Verification items for the finished model (mm, model axes). A direction names the side the tool comes from. Give positions to 0.01 mm unless a question says otherwise; leave off trailing zeros. Order: outer loops, then holes, each group sorted by start corner. A loop starts at its lowest first (then second) coordinate and runs counter-clockwise, first axis right, second up. Notation, with made-up numbers: (-26.5, 39.25) -> (19.5, 39.25) arc R14 cw to (19.5, 48.25) -> close; hole circle Ø3 at (-4, 17.25). An arc over 180 degrees is marked (long way). Write each question's results on one line, items separated by ' | '. Start each with the question number.
1. Mould release check, pull along X, two halves, no side actions. Record for faces 6 (the face through (-11.247, 0.143, 4.324)), 7 (the face through (-12, 0, 3)), 8 (the face through (0, 0, -3)), 9 (the face through (9.6, 0.07, 1.28)): +X half, -X half, draft (parallel to the pull), parting line (faces both ways), or undercut.
2. Cross-section at B-B, the plane x = -7.5. Enter the section's corners in (y, z), then the cut area to 3 significant figures.
3. Depth check by flat-ended pin: pin 1 Ø2 at (y, z) = (0.5, -2) entering from -X; pin 2 Ø3.5 at (x, y) = (-8, 0) entering from +Z; pin 3 Ø2.5 at (x, z) = (0, -1.5) entering from +Y. Enter the tip coordinate at first touch or a pass-through.
4. Material ranges on L1, parallel to X at y = -1.75, z = 4.5; L2, parallel to Z at x = -5.25, y = 0.25; L3, parallel to Y at x = 2.75, z = -1, recorded low to high. Write a range as from..to.
5. Cross-section at C-C, the plane z = 4.5. Enter the section's corners in (x, y).
6. Cross-section at A-A, the plane y = 0. Enter the section's corners in (x, z).
7. Set-up check for faces 1 (the face through (-6.6, -1.4, 2.6)), 2 (the face through (5, 0, -1)), 3 (the face through (-5, 0, -1)), 4 (the face through (0, -3, -1)), 5 (the face through (0, 3, -1)): record each of +Z, -Z, +X, -X, +Y, -Y from which the full face is reachable in a straight line by a thin tool's end or side.
8. Cross-section at D-D, the plane x = 9.25. Enter the section's corners in (y, z).
from build123d import *

# Parameters (mm, degrees)
BOSS_EXTRU_1_DEPTH                                 = 6
CHAMBRAGE_POUR_VIS_T_TE_HEXAGONALE_M31_D           = 3.2
CHAMBRAGE_POUR_VIS_T_TE_HEXAGONALE_M31_CBORE_D     = 6.5
CHAMBRAGE_POUR_VIS_T_TE_HEXAGONALE_M31_CBORE_DEPTH = 3.4
ESQUISSE6_W                                        = 10
ESQUISSE6_H                                        = 8
BOSS_EXTRU_2_DEPTH                                 = 3
CHANFREIN1_SIZE                                    = 0.2
ENL_V_MAT_EXTRU_5_REACH                            = 20.466
ESQUISSE10_W                                       = 3
ESQUISSE10_H                                       = 1


with BuildPart() as part:
    # Esquisse1 → Boss.-Extru.1 (new body)
    with BuildSketch(Plane.XY):
        with BuildLine():
            Line((-8, 4), (8, 4))
            ThreePointArc((8, 4), (12, 0), (8, -4))
            Line((8, -4), (-8, -4))
            ThreePointArc((-8, -4), (-12, 0), (-8, 4))
        make_face()
    extrude(amount=BOSS_EXTRU_1_DEPTH)

    # Chambrage pour vis à tête hexagonale M31 (through all)
    with Locations(Plane.XY.offset(6)):
        with Locations((-8, 0), (8, 0)):
            CounterBoreHole(CHAMBRAGE_POUR_VIS_T_TE_HEXAGONALE_M31_D / 2, CHAMBRAGE_POUR_VIS_T_TE_HEXAGONALE_M31_CBORE_D / 2, CHAMBRAGE_POUR_VIS_T_TE_HEXAGONALE_M31_CBORE_DEPTH)

    # Esquisse6 → Boss.-Extru.2 (add)
    with BuildSketch(Plane(origin=(0, 0, 0), x_dir=(-1, 0, 0), z_dir=(0, 0, -1))):
        Rectangle(ESQUISSE6_W, ESQUISSE6_H)
    extrude(amount=BOSS_EXTRU_2_DEPTH)

    # Chanfrein1
    chanfrein1_edges = [part.edges().sort_by_distance(p)[0] for p in [
        (5, 0, -3),
        (-5, 0, -3),
    ]]
    chamfer(chanfrein1_edges, length=CHANFREIN1_SIZE)

    # Esquisse10 → Enlèv. mat.-Extru.5 (cut, up to next)
    with BuildSketch(Plane(origin=(5, 0, 0), x_dir=(0, 0, -1), z_dir=(1, 0, 0)), mode=Mode.PRIVATE) as enl_v_mat_extru_5_sk1:
        with Locations((1.5, 3.5)):
            Rectangle(ESQUISSE10_W, ESQUISSE10_H)
    enl_v_mat_extru_5_tool1 = extrude(enl_v_mat_extru_5_sk1.sketch, amount=-ENL_V_MAT_EXTRU_5_REACH, mode=Mode.PRIVATE) & part.part
    # Esquisse10 → Enlèv. mat.-Extru.5 (cut, up to next)
    with BuildSketch(Plane(origin=(5, 0, 0), x_dir=(0, 0, -1), z_dir=(1, 0, 0)), mode=Mode.PRIVATE) as enl_v_mat_extru_5_sk2:
        with Locations((1.5, -3.5)):
            Rectangle(ESQUISSE10_W, ESQUISSE10_H)
    enl_v_mat_extru_5_tool2 = extrude(enl_v_mat_extru_5_sk2.sketch, amount=-ENL_V_MAT_EXTRU_5_REACH, mode=Mode.PRIVATE) & part.part
    add(enl_v_mat_extru_5_tool1.solids().sort_by_distance((5, 3.5, -1.5))[0], mode=Mode.SUBTRACT)
    add(enl_v_mat_extru_5_tool2.solids().sort_by_distance((5, -3.5, -1.5))[0], mode=Mode.SUBTRACT)


solid = part.part
Results below:
1) face 6: undercut | face 7: -X half | face 8: draft | face 9: undercut
2) outline: (-4, 0) -> (-1.52, 0) -> (-1.52, 2.6) -> (-3.21, 2.6) -> (-3.21, 6) -> (-4, 6) -> close; (1.52, 0) -> (4, 0) -> (4, 6) -> (3.21, 6) -> (3.21, 2.6) -> (1.52, 2.6) -> close | area: 18.3 mm²
3) pin 1: stops at x = -5 | pin 2: stops at z = 2.6 | pin 3: stops at y = 3
4) L1: x = -11.6..-10.74, -5.26..5.26, 10.74..11.6 | L2: z = 0..2.6 | L3: y = -3..3
5) outline: (-8, -4) -> (8, -4) arc R4 ccw to (8, 4) -> (-8, 4) arc R4 ccw to start; hole circle Ø6.5 at (-8, 0); hole circle Ø6.5 at (8, 0)
6) outline: (-12, 0) -> (-9.6, 0) -> (-9.6, 2.6) -> (-11.25, 2.6) -> (-11.25, 6) -> (-12, 6) -> close; (-6.4, 0) -> (-5, 0) -> (-5, -2.8) -> (-4.8, -3) -> (4.8, -3) -> (5, -2.8) -> (5, 0) -> (6.4, 0) -> (6.4, 2.6) -> (4.75, 2.6) -> (4.75, 6) -> (-4.75, 6) -> (-4.75, 2.6) -> (-6.4, 2.6) -> close; (9.6, 0) -> (12, 0) -> (12, 6) -> (11.25, 6) -> (11.25, 2.6) -> (9.6, 2.6) -> close
7) face 1: +Z | face 2: -Z, +X, +Y, -Y | face 3: -Z, -X, +Y, -Y | face 4: -Z, +X, -X, -Y | face 5: -Z, +X, -X, +Y
8) outline: (-3.8, 0) -> (-1, 0) -> (-1, 2.6) -> (-3, 2.6) -> (-3, 6) -> (-3.8, 6) -> close; (1, 0) -> (3.8, 0) -> (3.8, 6) -> (3, 6) -> (3, 2.6) -> (1, 2.6) -> close
